```python
from build123d import *

# Parameters (mm, degrees)
F2_W     = 6
F2_H     = 3
F3_DEPTH = 25
F4_R     = 1.5


with BuildPart() as f1:
    # F0 (on Front) → F1 (revolve)
    with BuildSketch(Plane.XZ):
        Polygon((-16.5, 2), (-14.5, 2), (-14.5, -11.4), (-12.5, -11.4), (-12.5, 2.059244), (0, 2.059244), (0, 4), (-16.5, 4), align=None)
    revolve(axis=Axis((0, 0, -8.009328), (0, 0, -1)))

    # F2 (on face) → F3 (cut)
    with BuildSketch(Plane.XY.offset(4)):
        Rectangle(F2_W, F2_H)
    extrude(amount=-F3_DEPTH, mode=Mode.SUBTRACT)

    # F4
    f4_edges = [f1.edges().sort_by_distance(p)[0] for p in [
        (16.5, 0, 4),
    ]]
    fillet(f4_edges, radius=F4_R)


solid = f1.part
```
The listing builds one solid part. Answer for the finished solid, in the listing's coordinates (mm). A direction names the side the tool comes from. Give positions to 0.01 mm unless a question says otherwise; leave off trailing zeros. Order: outer loops, then holes, each group sorted by start corner. A loop starts at its lowest first (then second) coordinate and runs counter-clockwise, first axis right, second up. Notation, with made-up numbers: (52.25, -22.75) -> (107.25, -22.75) arc R6 ccw to (107.25, -18.75) -> close; hole circle Ø9 at (-22.5, 42.25). An arc over 180 degrees is marked (long way). Answer as a JSON object with one key per item and string values. Group by question number.
Item 1: The part is cut by section B-B on x = 0. Write down the section's boundary in (y, z).
Item 2: Flat-ended cylindrical pins translate along their axes: pin 1 (1.5 mm diameter, centred on x = -1.5, z = -6, fed in from +Y); pin 2 (2 mm diameter, centred on x = 13, z = -4, fed in from -Y); pin 3 (1 mm diameter, centred on y = 0.5, z = 3.5, fed in from +X); pin 4 (2 mm diameter, centred on x = -1, z = 3, fed in from -Y). Find the tip coordinate at first contact, or state that the pin passes through.
Item 3: A tool of negligible diameter and unlimited length cuts with its end or side. For faces 1 (the flat face through (0, -3, 2.059)), 2 (the flat face through (0, -3, 4)), 3 (the flat face through (0, -1.5, 3)), from which of +Z, -Z, +X, -X, +Y, -Y can it reach the whole face along a straight path? Write none if from no direction.
Item 4: The part is cut by section A-A on y = 0. Write down the section's boundary in (x, z).
Item 5: The part is cut by section C-C on z = -4. Write down the section's boundary in (x, y).
Item 6: Consider L1, parallel to Y at x = 0, z = -3; L2, parallel to Z at x = 2, y = -2; L3, parallel to Z at x = 13, y = -7.5. Determine where each line is inside the solid, lowest interval first. Write a range as from..to.
Item 7: Determine the mould class of faces 4 (the flat face through (0, -15, 2)), 5 (the flat face through (-3, 0, 3)), 6 (the flat face through (3, 0, 3)), 7 (the cylindrical face through (-6.691, -12.864, -4.794)) for opening direction Y: pulls with the +Y half, pulls with the -Y half, needs draft (parallel to the pull), parting line crosses it, or undercut.
Result set:
{
 "1": {"outline": "(-16.5, 2) -> (-14.5, 2) -> (-14.5, -11.4) -> (-12.5, -11.4) -> (-12.5, 2.06) -> (-1.5, 2.06) -> (-1.5, 4) -> (-15, 4) arc R1.5 ccw to (-16.5, 2.5) -> close; (1.5, 2.06) -> (12.5, 2.06) -> (12.5, -11.4) -> (14.5, -11.4) -> (14.5, 2) -> (16.5, 2) -> (16.5, 2.5) arc R1.5 ccw to (15, 4) -> (1.5, 4) -> close"},
 "2": {"pin 1": "y = 14.48", "pin 2": "y = -8.14", "pin 3": "x = 16.41", "pin 4": "y = -16.5"},
 "3": {"face 1": "-Z", "face 2": "+Z, +X, -X, +Y, -Y", "face 3": "+Z, -Z"},
 "4": {"outline": "(-16.5, 2) -> (-14.5, 2) -> (-14.5, -11.4) -> (-12.5, -11.4) -> (-12.5, 2.06) -> (-3, 2.06) -> (-3, 4) -> (-15, 4) arc R1.5 ccw to (-16.5, 2.5) -> close; (3, 2.06) -> (12.5, 2.06) -> (12.5, -11.4) -> (14.5, -11.4) -> (14.5, 2) -> (16.5, 2) -> (16.5, 2.5) arc R1.5 ccw to (15, 4) -> (3, 4) -> close"},
 "5": {"outline": "circle Ø29 at (0, 0); hole circle Ø25 at (0, 0)"},
 "6": {"L1": "-14.5..-12.5, 12.5..14.5", "L2": "2.06..4", "L3": "2..4"},
 "7": {"face 4": "needs draft", "face 5": "undercut", "face 6": "undercut", "face 7": "parting line crosses it"}
}
